```python
from build123d import *

# Parameters (mm, degrees)
SKETCH1_R           = 25
SKETCH1_R_2         = 12.5
BOSS_EXTRUDE1_DEPTH = 17.5
BOSS_EXTRUDE2_DEPTH = 25
CUT_EXTRUDE1_START  = -50
SKETCH3_R           = 12.5
CUT_EXTRUDE1_DEPTH  = 50
BOSS_EXTRUDE3_DEPTH = 25
SKETCH5_W           = 10
SKETCH5_H           = 75.978198428
CUT_EXTRUDE2_DEPTH  = 5
SKETCH6_R           = 5
CUT_EXTRUDE3_DEPTH  = 101.657736852


with BuildPart() as part:
    # Sketch1 → Boss-Extrude1 (new, symmetric)
    with BuildSketch(Plane(origin=(0, 0, 0), x_dir=(1, 0, 0), z_dir=(0, 1, 0))):
        with Locations(Location((0, 0, 0), (0, 0, 270))):
            Circle(SKETCH1_R)
        with Locations(Location((0, 0, 0), (0, 0, 270))):
            Circle(SKETCH1_R_2, mode=Mode.SUBTRACT)
    extrude(amount=BOSS_EXTRUDE1_DEPTH, both=True)

    # Sketch2 → Boss-Extrude2 (add, symmetric)
    with BuildSketch(Plane.XY):
        Polygon((-15, 7.5), (-50, 7.5), (-50, -7.5), (-15, -7.5), (0, -7.5), (0, 7.5), align=None)
    extrude(amount=BOSS_EXTRUDE2_DEPTH, both=True)

    # Sketch3 → Cut-Extrude1 (cut)
    with BuildSketch(Plane(origin=(0, 17.5, 0), x_dir=(1, 0, 0), z_dir=(0, 1, 0)).offset(CUT_EXTRUDE1_START)):
        with Locations(Location((0, 0, 0), (0, 0, 270))):
            Circle(SKETCH3_R)
    extrude(amount=CUT_EXTRUDE1_DEPTH, mode=Mode.SUBTRACT)

    # Sketch4 → Boss-Extrude3 (add, symmetric)
    with BuildSketch(Plane.XY):
        Polygon((-50, 7.5), (-94.271090497, -15.73941794), (-86.771090497, -28.729798997), (-50, -7.5), align=None)
    extrude(amount=BOSS_EXTRUDE3_DEPTH, both=True)

    # Sketch5 → Cut-Extrude2 (cut)
    with BuildSketch(Plane(origin=(-13.887914048, 26.456475856, 0), x_dir=(0.8854218099422688, 0.4647883588027534, 0), z_dir=(-0.4647883588027534, 0.8854218099422688, 0))):
        with Locations((-65.785177806, 0)):
            Rectangle(SKETCH5_W, SKETCH5_H)
    extrude(amount=-CUT_EXTRUDE2_DEPTH, mode=Mode.SUBTRACT)

    # Sketch6 → Cut-Extrude3 (cut, through all)
    with BuildSketch(Plane(origin=(-13.887914048, 26.456475856, 0), x_dir=(0.8854218099422688, 0.4647883588027534, 0), z_dir=(-0.4647883588027534, 0.8854218099422688, 0))):
        with Locations(Location((-80.785177806, 0, 0), (0, 0, 180))):
            Circle(SKETCH6_R)
    extrude(amount=-CUT_EXTRUDE3_DEPTH, mode=Mode.SUBTRACT)


solid = part.part
```
Build history of the part. All positions in model axes, mm. A direction names the side the tool comes from. Coordinates: 2 decimals unless noted, no trailing zeros. Write each loop counter-clockwise with the first axis right and the second up, starting at its lowest first coordinate (ties: lowest second). Pieces come first, ordered by that corner, then holes.
1. Band-saw the part on B-B, the plane x = 9. Give the cut face in (y, z).
Answer block:
outline: (-17.5, -23.32) - (17.5, -23.32) - (17.5, -8.67) - (-17.5, -8.67) - close; (-17.5, 8.67) - (17.5, 8.67) - (17.5, 23.32) - (-17.5, 23.32) - close
2. 3-axis set-ups, long thin cutter, end or side, ignore diameter. For faces 5 (the flat face through (-66.56, -3.98, 0.35)), 6 (the flat face through (-75.417, -8.626, 0.35)), 7 (the flat face through (-68.64, -18.26, 0.35)), 8 (the flat face through (-36, 7.5, 0)): which of +Z, -Z, +X, -X, +Y, -Y reach the whole face in a straight line?
Answer block:
face 5: +Z, -Z, -X
face 6: +Z, -Z, +Y
face 7: +Z, -Z, -Y
face 8: -X, +Y
3. Drop flat-ended pins along their axis: pin 1 (10 mm diameter, centred on x = -20, y = 12, fed in from +Z); pin 2 (8 mm diameter, centred on x = -74, z = 11, fed in from +Y); pin 3 (1.5 mm diameter, centred on x = 4, y = 8, fed in from -Z); pin 4 (3 mm diameter, centred on x = -41, z = -1.5, fed in from -Y). Give the stop position or say it passes through.
Answer block:
pin 1: stops at z = 25
pin 2: stops at y = -6.44
pin 3: stops at z = -24.79
pin 4: stops at y = -7.5
4. Band-saw the part on D-D, the plane z = 0. Give the cut face in (x, y), and give its area (3 significant figures).
Answer block:
outline: (-94.27, -15.74) - (-86.77, -28.73) - (-82.96, -26.53) - (-89.84, -13.42) - close; (-80.99, -8.77) - (-74.29, -21.53) - (-50, -7.5) - (-25, -7.5) - (-25, -17.5) - (-12.5, -17.5) - (-12.5, 17.5) - (-25, 17.5) - (-25, 7.5) - (-50, 7.5) - (-67.71, -1.8) - (-65.38, -6.22) - (-74.24, -10.87) - (-76.56, -6.44) - close; (12.5, -17.5) - (25, -17.5) - (25, 17.5) - (12.5, 17.5) - close
area: 1,700 mm2
5. Pull direction Z, two halves, no side cores. Call faces 1 (the flat face through (-48, -6, 25)), 2 (the cylindrical face through (-77.6, -15.235, 0.22)), 3 (the cylindrical face through (3.755, -0.245, 11.923)), 4 (the flat face through (-90.6, -22.1, 0.4)): released by +Z, released by -Z, zero draft, split by the parting line, or undercut.
Answer block:
face 1: released by +Z
face 2: undercut
face 3: undercut
face 4: zero draft
6. Band-saw the part on A-A, the plane z = -9. Give the cut face in (x, y), and give its area (3 significant figures).
Answer block:
outline: (-94.27, -15.74) - (-86.77, -28.73) - (-50, -7.5) - (-23.32, -7.5) - (-23.32, -17.5) - (-8.67, -17.5) - (-8.67, 17.5) - (-23.32, 17.5) - (-23.32, 7.5) - (-50, 7.5) - (-67.71, -1.8) - (-65.38, -6.22) - (-74.24, -10.87) - (-76.56, -6.44) - close; (8.67, -17.5) - (23.32, -17.5) - (23.32, 17.5) - (8.67, 17.5) - close
area: 2,030 mm2
7. Drill centre lines: probe 1 along X at (y, z) = (-9, 0); probe 2 along X at (y, z) = (8, 0); probe 3 along Y at (x, z) = (4, -12). Where is each one in solid material? Low to high.
Answer block:
probe 1: x = -80.87 to -75.22, -70.67 to -52.6, -25 to -12.5, 12.5 to 25
probe 2: x = -25 to -12.5, 12.5 to 25
probe 3: y = -17.5 to 17.5
8. Band-saw the part on C-C, the plane y = 1.5. Give the cut face in (x, z).
Answer block:
outline: (-61.43, -25) - (0, -25) arc R25 ccw to (0, 25) - (-61.43, 25) - close; hole circle Ø25 at (0, 0)
